The listing builds one solid part. Answer for the finished solid, in the listing's coordinates (mm). Coordinates: 2 decimals unless noted, no trailing zeros. Loops run counter-clockwise (first coordinate to the right, second up) from the corner with the lowest first, then second, coordinate; pieces in that order, holes last. Notation, with made-up numbers: (69.25, 78.5) - (116.25, 78.5) arc R10 ccw to (116.25, 88.5) - close; hole circle Ø6 at (33.25, 30). An arc over 180 degrees is marked (long way). Use one line per item in the form item = value. Start each with the question number.
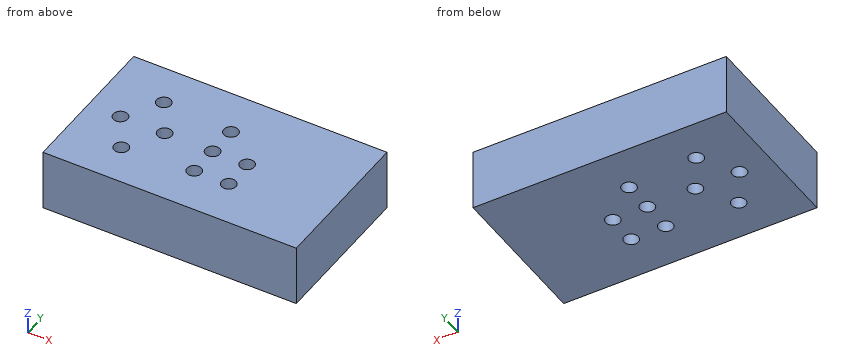
```python
from build123d import *

# Parameters (mm, degrees)
SKETCH1_W           = 132
SKETCH1_H           = 79
BOSS_EXTRUDE2_DEPTH = 32
SKETCH1_6_R         = 3.75
CUT_EXTRUDE15_DEPTH = 42


with BuildPart() as part:
    # Sketch1 → Boss-Extrude2 (new body)
    with BuildSketch(Plane.XY):
        with Locations((-7.24491948, 0)):
            Rectangle(SKETCH1_W, SKETCH1_H)
    extrude(amount=BOSS_EXTRUDE2_DEPTH)

    # Sketch1_6 → Cut-Extrude15 (cut)
    with BuildSketch(Plane.XY):
        with Locations(Location((-45, 18.5, 0), (0, 0, 180))):
            Circle(SKETCH1_6_R)
        with Locations(Location((-45, -18.5, 0), (0, 0, 180))):
            Circle(SKETCH1_6_R)
        with Locations(Location((-56.5, 0, 0), (0, 0, 180))):
            Circle(SKETCH1_6_R)
        with Locations(Location((-33.5, 0, 0), (0, 0, 180))):
            Circle(SKETCH1_6_R)
        with Locations(Location((-8.5, 0, 0), (0, 0, 180))):
            Circle(SKETCH1_6_R)
        with Locations(Location((-8.5, -16, 0), (0, 0, 180))):
            Circle(SKETCH1_6_R)
        with Locations(Location((-8.5, 16, 0), (0, 0, 180))):
            Circle(SKETCH1_6_R)
        with Locations(Location((9.5, -16, 0), (0, 0, 180))):
            Circle(SKETCH1_6_R)
        with Locations(Location((9.5, 0, 0), (0, 0, 180))):
            Circle(SKETCH1_6_R)
    extrude(amount=CUT_EXTRUDE15_DEPTH, mode=Mode.SUBTRACT)


solid = part.part
```
(1) A cutting plane is placed at A-A (x = 9.5). Determine the outline of the cut face in (y, z).
(2) Find the intervals of material crossed by probe 1 along Y at (x, z) = (9.5, 24); probe 2 along Y at (x, z) = (-8.5, 7.5); probe 3 along Y at (x, z) = (-45, 15), in increasing order. Write a range as from..to.
(3) A cutting plane is placed at B-B (z = 13). State how many separate pieces and enclosed holes the cut face has, then the cut area to 3 significant figures.
(4) A cutting plane is placed at C-C (x = -33.5). Determine the outline of the cut face in (y, z), then the cut area to 3 significant figures.
(5) A cutting plane is placed at D-D (x = -8.5). Determine the outline of the cut face in (y, z).
Evaluation:
q1.outline = (-39.5, 0) - (-19.75, 0) - (-19.75, 32) - (-39.5, 32) - close; (-12.25, 0) - (-3.75, 0) - (-3.75, 32) - (-12.25, 32) - close; (3.75, 0) - (39.5, 0) - (39.5, 32) - (3.75, 32) - close
q2.probe_1 = -39.5..-19.75, -12.25..-3.75, 3.75..39.5
q2.probe_2 = -39.5..-19.75, -12.25..-3.75, 3.75..12.25, 19.75..39.5
q2.probe_3 = -39.5..-22.25, -14.75..14.75, 22.25..39.5
q3.separate_pieces = 1
q3.enclosed_holes = 9
q3.area = 10,000 mm^2
q4.outline = (-39.5, 0) - (-3.75, 0) - (-3.75, 32) - (-39.5, 32) - close; (3.75, 0) - (39.5, 0) - (39.5, 32) - (3.75, 32) - close
q4.area = 2,290 mm^2
q5.outline = (-39.5, 0) - (-19.75, 0) - (-19.75, 32) - (-39.5, 32) - close; (-12.25, 0) - (-3.75, 0) - (-3.75, 32) - (-12.25, 32) - close; (3.75, 0) - (12.25, 0) - (12.25, 32) - (3.75, 32) - close; (19.75, 0) - (39.5, 0) - (39.5, 32) - (19.75, 32) - close
